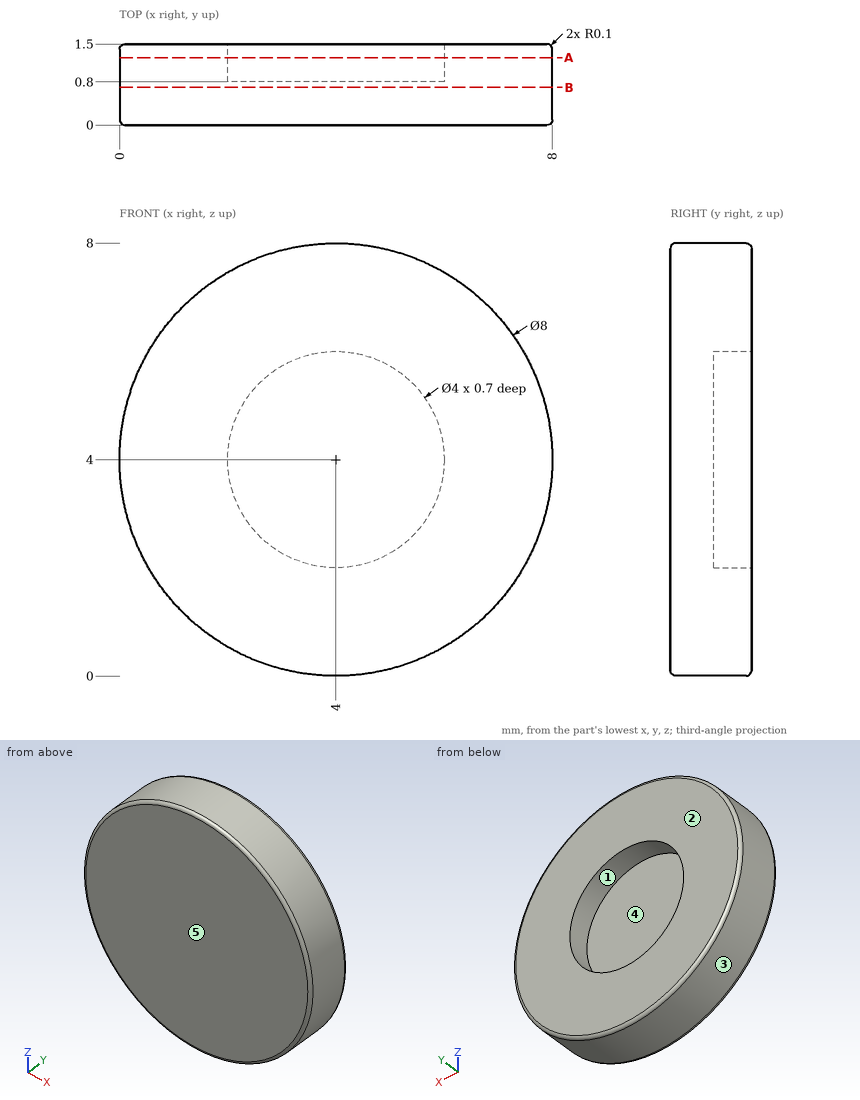
Geometry: see drawing. Coordinates: mm, zero at the bounding-box minimum. A direction names the side the tool comes from. Give positions to 0.01 mm unless a question says otherwise; leave off trailing zeros. Order: outer loops, then holes, each group sorted by start corner. A loop starts at its lowest first (then second) coordinate and runs counter-clockwise, first axis right, second up. Notation, with made-up numbers: (73.25, 26) -> (127.25, 26) arc R14 ccw to (127.25, 41) -> close; hole circle Ø4 at (-19, -18). An arc over 180 degrees is marked (long way). Write item = value, one per line.
Q1. Set-up query: the marked faces 4 and 5. Return all of +Z, -Z, +X, -X, +Y, -Y with unobstructed straight access to the full face (end or side cutting, diameter ignored); none if empty.
Data:
face_4 = +Y
face_5 = +Z, -Z, +X, -X, -Y
Q2. Material intervals for line 1 (Z direction, x = 4, y = 1.1); line 2 (Y direction, x = 4.5, z = 2.5); line 3 (X direction, y = 1.3, z = 3.5), sorted ascending. Write a range as from..to.
Data:
line_1 = 0..2, 6..8
line_2 = 0..0.8
line_3 = 0.03..2.06, 5.94..7.97
Q3. Pull-direction query (Z, two-part tool) for the marked faces 1, 2 and 3; classes: released by +Z, released by -Z, zero draft, split by the parting line, or undercut.
Data:
face_1 = undercut
face_2 = zero draft
face_3 = split by the parting line
Q4. Cut plane B-B, the plane y = 0.7. Output: boundary loops of the cut face in (x, z), and give its area (3 significant figures).
Data:
outline = circle Ø8 at (4, 4)
area = 50.3 mm^2
Q5. Cut plane A-A, the plane y = 1.25. Output: boundary loops of the cut face in (x, z), and give its area (3 significant figures).
Data:
outline = circle Ø8 at (4, 4); hole circle Ø4 at (4, 4)
area = 37.7 mm^2
